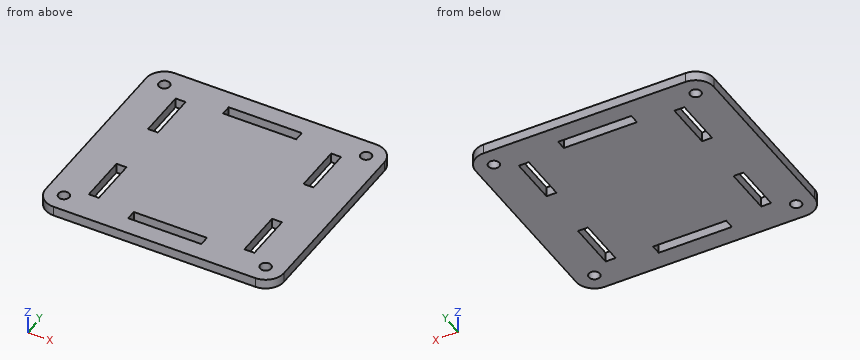
from build123d import *

# Parameters (mm, degrees)
SKETCH_1_W         = 88
SKETCH_1_H         = 98
SKETCH_1_W_2       = 4.1
SKETCH_1_H_2       = 30.1
SKETCH_1_W_3       = 20.1
SKETCH_1_H_3       = 4.1
EXTRUDE_1_DEPTH    = 4
HOLE_WIZARD_M4_1_D = 4.5
FILLET_3_R         = 7.5


with BuildPart() as part:
    # ｽｹｯﾁ1 → ﾎﾞｽ - 押し出し1 (new body)
    with BuildSketch(Plane(origin=(0, 0, 0), x_dir=(0, 1, 0), z_dir=(0, 0, 1))):
        with Locations((44, 49)):
            Rectangle(SKETCH_1_W, SKETCH_1_H)
        with Locations((78.5, 49)):
            Rectangle(SKETCH_1_W_2, SKETCH_1_H_2, mode=Mode.SUBTRACT)
        with Locations((22.5, 81)):
            Rectangle(SKETCH_1_W_3, SKETCH_1_H_3, mode=Mode.SUBTRACT)
        with Locations((65.5, 81)):
            Rectangle(SKETCH_1_W_3, SKETCH_1_H_3, mode=Mode.SUBTRACT)
        with Locations((22.5, 17)):
            Rectangle(SKETCH_1_W_3, SKETCH_1_H_3, mode=Mode.SUBTRACT)
        with Locations((65.5, 17)):
            Rectangle(SKETCH_1_W_3, SKETCH_1_H_3, mode=Mode.SUBTRACT)
        with Locations((9.5, 49)):
            Rectangle(SKETCH_1_W_2, SKETCH_1_H_2, mode=Mode.SUBTRACT)
    extrude(amount=EXTRUDE_1_DEPTH)

    # M4 すきま穴1 (through all)
    with Locations(Plane.XY.offset(4)):
        with Locations((-90.5, 80.5), (-7.5, 80.5), (-7.5, 7.5), (-90.5, 7.5)):
            Hole(HOLE_WIZARD_M4_1_D / 2)

    # ﾌｨﾚｯﾄ3
    fillet_3_edges = [part.edges().sort_by_distance(p)[0] for p in [
        (-98, 0, 2),
        (-98, 88, 2),
        (0, 88, 2),
        (0, 0, 2),
    ]]
    fillet(fillet_3_edges, radius=FILLET_3_R)


solid = part.part
For this review, take the finished solid that the model builds, in its own axes (mm). Give positions to 0.01 mm unless a question says otherwise; leave off trailing zeros. Order: outer loops, then holes, each group sorted by start corner. A loop starts at its lowest first (then second) coordinate and runs counter-clockwise, first axis right, second up. Notation, with made-up numbers: (34, -28) - (84, -28) arc R32 ccw to (84, 6) - close; hole circle Ø6 at (49.5, 83). An arc over 180 degrees is marked (long way). Answer as a JSON object with one key per item and string values. Group by question number.
Item 1: Take a section at A-A on y = 24. Give the boundary of the cut face in (x, z).
Item 2: Take a section at B-B on x = -55. Give the boundary of the cut face in (y, z).
Item 3: Wall thickness on line 1 along X through (y, z) = (20, 0.45); line 2 along Y through (x, z) = (-48, 3.15); line 3 along Y through (x, z) = (-19, 0.8): over which ranges is each line inside the solid? List them lowest first.
Item 4: Take a section at C-C on z = 1.55. Give the number of separate pieces and of enclosed holes in the cut face, and give its area (3 significant figures).
Item 5: Clearance check with a flat-ended pin moving along its axis: pin 1 Ø2.5 at (x, y) = (-90.5, 80.5) entering from +Z. State where the tip first meets the part, or that it passes through.
Reported:
{
 "1": {"outline": "(-98, 0) - (-83.05, 0) - (-83.05, 4) - (-98, 4) - close; (-78.95, 0) - (-19.05, 0) - (-19.05, 4) - (-78.95, 4) - close; (-14.95, 0) - (0, 0) - (0, 4) - (-14.95, 4) - close"},
 "2": {"outline": "(0, 0) - (7.45, 0) - (7.45, 4) - (0, 4) - close; (11.55, 0) - (76.45, 0) - (76.45, 4) - (11.55, 4) - close; (80.55, 0) - (88, 0) - (88, 4) - (80.55, 4) - close"},
 "3": {"line 1": "-98 to -83.05, -78.95 to -19.05, -14.95 to 0", "line 2": "0 to 7.45, 11.55 to 76.45, 80.55 to 88", "line 3": "0 to 12.45, 32.55 to 55.45, 75.55 to 88"},
 "4": {"separate pieces": "1", "enclosed holes": "10", "area": "7,940 mm^2"},
 "5": {"pin 1": "through"}
}
